Part model, mm, in its own coordinate system. A direction names the side the tool comes from. Give positions to 0.01 mm unless a question says otherwise; leave off trailing zeros. Order: outer loops, then holes, each group sorted by start corner. A loop starts at its lowest first (then second) coordinate and runs counter-clockwise, first axis right, second up. Notation, with made-up numbers: M 39,-22.75 L 60,-22.75 A24 ccw 60,-3.75 Z; hole C 6,74 d10. An arc over 180 degrees is marked long. One line per question, with ' | ' between items.
Autodesk Inventor part; units mm, degrees
ref_plane "YZ Plane" through (0, 0, 0) normal (1, 0, 0) x (0, 1, 0)
ref_plane "XZ Plane" through (0, 0, 0) normal (0, 1, 0) x (-1, 0, 0)
sketch "Skizze1" plane through (0, 0, 0) normal (0, 0, 1) x (1, 0, 0)
  circle A0 centre (0, 0) radius 5
  dimension "d0" = 10
extrude "Extrusion1" add sketch "Skizze1" along normal blind 20
sketch "Skizze6" plane through (0, 0, 0) normal (0, 0, -1) x (-1, 0, 0)
  circle A0 centre (0, 0) radius 5
  circle A1 centre (0, 0) radius 2.5
  dimension "d25" = 5
extrude "Extrusion6" add sketch "Skizze6" along normal blind 10 contours A1
ref_plane "Arbeitsebene3" through (0, 0, 10) normal (0, 0, 1) x (1, 0, 0)
mirror "Spiegeln2" about plane through (0, 0, 10) normal (0, 0, 1) of "Extrusion6"
equation "\"d0\" = Durchmesser3"
equation "\"Durchmesser1\" = 15"
equation "\"Größe1\" = 7"
equation "\"Durchmesser2\" = 3"
equation "\"Durchmesser3\" = 10"
equation "\"Größe3\" = 3"
equation "\"Größe4\" = 15"
properties part number "WellenSchiffsschraube2"
1. Slice it at D-D on z = 26. Give the cut face in (x, y), then the cut area to 3 significant figures.
Worked out:
outline: C 0,0 d5 | area: 19.6 mm2
2. Drop flat-ended pins along their axis: pin 1 (5 mm diameter, centred on x = 0.5, z = -4, fed in from -Y); pin 2 (1 mm diameter, centred on x = -1, z = 2.5, fed in from -Y); pin 3 (5 mm diameter, centred on y = 3, z = 8.5, fed in from +X). Give the stop position or say it passes through.
Worked out:
pin 1: stops at y = -2.5 | pin 2: stops at y = -4.97 | pin 3: stops at x = 4.97
3. Slice it at C-C on z = 0.5. Give the cut face in (x, y), then the cut area to 3 significant figures.
Worked out:
outline: C 0,0 d10 | area: 78.5 mm2
4. Probe L1, parallel to Z at x = 0, y = -3; L2, parallel to X at y = -0.25, z = 7; L3, parallel to Y at x = 0, z = 25. List the from-to ranges inside material, lowest first. Write a range as from..to.
Worked out:
L1: z = 0..20 | L2: x = -4.99..4.99 | L3: y = -2.5..2.5
5. Slice it at A-A on x = 0. Give the cut face in (y, z), then the cut area to 3 significant figures.
Worked out:
outline: M -5,0 L -2.5,0 L -2.5,-10 L 2.5,-10 L 2.5,0 L 5,0 L 5,20 L 2.5,20 L 2.5,30 L -2.5,30 L -2.5,20 L -5,20 Z | area: 300 mm2
6. Tool access for faces 1 (the flat face through (2, -2, 20)), 2 (the cylindrical face through (0.54, 2.44, -4.93)), 3 (the flat face through (0, 0, 30)): list every direction of +Z, -Z, +X, -X, +Y, -Y with a clear straight run to the whole face (end or side of a thin tool).
Worked out:
face 1: +Z | face 2: -Z | face 3: +Z, +X, -X, +Y, -Y
